Autodesk Inventor part; units mm, degrees
ref_plane "YZ Plane" through (0, 0, 0) normal (1, 0, 0) x (0, 1, 0)
ref_plane "XZ Plane" through (0, 0, 0) normal (0, 1, 0) x (-1, 0, 0)
ref_plane "XY Plane" through (0, 0, 0) normal (0, 0, 1) x (1, 0, 0)
sketch "草圖1" plane through (0, 0, 0) normal (0, 1, 0) x (-1, 0, 0)
  arc A0 (-45, 0) -> (0, -45) centre (0, 0) ccw construction
  arc A1 (-67.5, 0) -> (0, -67.5) centre (0, 0) ccw
  arc A2 (-22.5, 0) -> (0, -22.5) centre (0, 0) ccw
  arc A3 (-22.5, 0) -> (-67.5, 0) centre (-45, 0) ccw
  arc A4 (0, -22.5) -> (0, -67.5) centre (0, -45) ccw
  dimension "d1" = 45
  dimension "d3" = 22.5
extrude "擠出1" add sketch "草圖1" along normal blind 4
sketch "草圖3" plane through (0, 0, 0) normal (0, -1, 0) x (1, 0, 0)
  arc A0 (0, -45) -> (45, 0) centre (0, 0) ccw construction
  line L0 (45, 0) -> (31.3889, -32.245)
  dimension "d7" = 35
hole "孔1" at (45, 0, 0) at (31.3889, 0, -32.245) direction (0, 1, 0) diameter 2.459 end through all
properties part number "A0004"
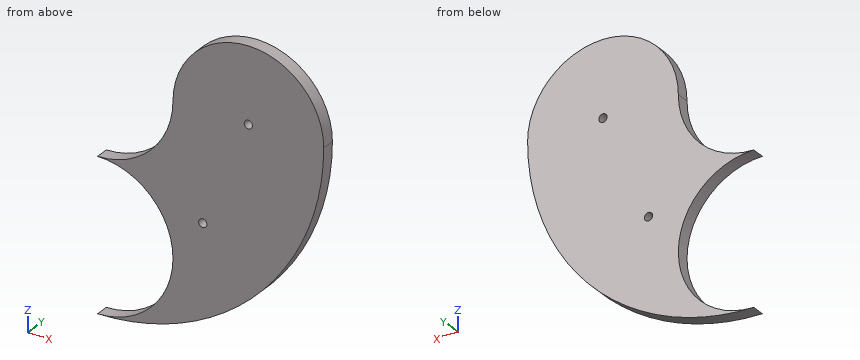
Work out the finished part from the listing and answer in its coordinate system (mm). Coordinates: 2 decimals unless noted, no trailing zeros. Loops run counter-clockwise (first coordinate to the right, second up) from the corner with the lowest first, then second, coordinate; pieces in that order, holes last. Notation, with made-up numbers: (-31.75, -30.5) -> (27.25, -30.5) arc R14 cw to (27.25, -22.5) -> close; hole circle Ø6 at (21, 69). An arc over 180 degrees is marked (long way). Write each question's results on one line, items separated by ' | '. Start each with the question number.
1) Find section C-C on z = 13.5. Determine the outline of the cut face in (x, y).
2) Consider line 1 along X through (y, z) = (3.1, 0); line 2 along Z through (x, y) = (9.5, 3.15); line 3 along Z through (x, y) = (19, 1.8). Determine where each line is inside the solid, lowest interval first.
3) Find section D-D on x = 13. Determine the outline of the cut face in (y, z).
4) Find section B-B on y = 2. Determine the outline of the cut face in (x, z) (1 decimal).
5) Find section A-A on x = 45. Determine the outline of the cut face in (y, z).
6) Flat-ended cylindrical pins translate along their axes: P1, Ø1.5, axis at x = 9.5, y = 2, coming from the -Z side; P2, Ø1, axis at x = 42, y = 0.5, coming from the -Z side. Find the tip coordinate at first contact, or state that the pin passes through.
Response values:
1) outline: (27, 0) -> (63, 0) -> (63, 4) -> (27, 4) -> close
2) line 1: x = 22.5 to 43.77, 46.23 to 67.5 | line 2: z = -66.83 to -65.4, -24.6 to -20.4 | line 3: z = -64.77 to -57.05, -32.95 to -12.05
3) outline: (0, -66.24) -> (4, -66.24) -> (4, -63.36) -> (0, -63.36) -> close; (0, -26.64) -> (4, -26.64) -> (4, -18.36) -> (0, -18.36) -> close
4) outline: (0, -67.5) arc R67.5 ccw to (67.5, 0) arc R22.5 ccw to (22.5, 0) arc R22.5 cw to (0, -22.5) arc R22.5 cw to start; hole circle Ø2.5 at (31.4, -32.2); hole circle Ø2.5 at (45, 0)
5) outline: (0, -50.31) -> (4, -50.31) -> (4, -1.23) -> (0, -1.23) -> close; (0, 1.23) -> (4, 1.23) -> (4, 22.5) -> (0, 22.5) -> close
6) P1: stops at z = -66.93 | P2: stops at z = -53.24
